from build123d import *

# Parameters (mm, degrees)
F0_W     = 140
F0_H     = 34.5
F1_DEPTH = 96
F2_W     = 140
F2_H     = 14.5
F3_DEPTH = 88
F4_W     = 1.7
F4_H     = 35.4929193519
F4_W_2   = 15.0318985057
F4_H_2   = 10
F5_DEPTH = 88


with BuildPart() as f1:
    # F0 (on Top) → F1 (new body)
    with BuildSketch(Plane.XY):
        with Locations((41.4941184592, -5.2499999292)):
            Rectangle(F0_W, F0_H)
    extrude(amount=F1_DEPTH)

    # F2 (on face) → F3 (cut)
    with BuildSketch(Plane.XY.offset(96)):
        with Locations((41.4941184592, -5.2499999292)):
            Rectangle(F2_W, F2_H)
    extrude(amount=-F3_DEPTH, mode=Mode.SUBTRACT)

    # F4 (on face) → F5 (cut)
    with BuildSketch(Plane.XY.offset(96)):
        Polygon((-13.0666754805, 12.0000000708), (-15.4708385365, 12.0000000708), (20.0220808154, -23.4929192811), (22.4262438715, -23.4929192811), align=None)
        Polygon((81.1649545925, 12.0000000708), (78.7607915364, 12.0000000708), (42.6027141511, -24.1580773145), (45.0068772072, -24.1580773145), align=None)
        with Locations((33.3644790113, -5.7464596052)):
            Rectangle(F4_W, F4_H)
        with Locations((103.9781692064, 7.0000000708)):
            Rectangle(F4_W_2, F4_H_2)
    extrude(amount=-F5_DEPTH, mode=Mode.SUBTRACT)


solid = f1.part
Verification items for the finished model (mm, model axes). A direction names the side the tool comes from. Give positions to 0.01 mm unless a question says otherwise; leave off trailing zeros. Write each loop counter-clockwise with the first axis right and the second up, starting at its lowest first coordinate (ties: lowest second). Pieces come first, ordered by that corner, then holes. Notation, with made-up numbers: (2, 31.5) - (39, 31.5) arc R14 ccw to (39, 56.5) - close; hole circle Ø5 at (62.25, 18.25). An arc over 180 degrees is marked (long way). Answer as CSV lines item,"result". Start each with the question number.
1. Draft check along X on faces 1 (the face through (9, 7, 96)), 2 (the face through (-7.997, 6.93, 52.616)). Enter one of: pulls with the +X half, pulls with the -X half, needs draft (parallel to the pull), parting line crosses it, or undercut.
2. Sectioned sample at C-C (y = 4.5). Record the boundary of the cut face in (x, z), then the cut area to 3 significant figures.
3. Thickness scan on line 1 (Y direction, x = 42, z = 73); line 2 (Y direction, x = 77, z = 87); line 3 (X direction, y = 5.5, z = 43.5). Record the ranges inside material, lowest first.
4. Sectioned sample at A-A (z = 28). Count the separate pieces of the cut face and the enclosed holes in it, then the cut area to 3 significant figures.
5. Set-up check for faces 3 (the face through (32.514, 7, 53)), 4 (the face through (51.595, -17.57, 52.616)), 5 (the face through (56, 7, 96)), 6 (the face through (84, -12.5, 53)), 7 (the face through (41, 12, 47)): record each of +Z, -Z, +X, -X, +Y, -Y from which the full face is reachable in a straight line by a thin tool's end or side.
6. Sectioned sample at D-D (x = 99.5). Record the boundary of the cut face in (y, z).
7. Depth check by flat-ended pin: pin 1 (3 mm diameter, centred on y = 4.5, z = 34, fed in from +X). Enter the tip coordinate at first touch or a pass-through.
8. Sectioned sample at B-B (x = 4). Record the boundary of the cut face in (y, z), then the cut area to 3 significant figures.
Derived:
1,face 1,"needs draft"
1,face 2,"undercut"
2,outline,"(-28.51, 0) - (111.49, 0) - (111.49, 8) - (96.46, 8) - (96.46, 96) - (73.66, 96) - (73.66, 8) - (71.26, 8) - (71.26, 96) - (34.21, 96) - (34.21, 8) - (32.51, 8) - (32.51, 96) - (-5.57, 96) - (-5.57, 8) - (-7.97, 8) - (-7.97, 96) - (-28.51, 96) - close"
2,area,"11,500 mm²"
3,line 1,"-22.5 to -12.5, 2 to 12"
3,line 2,"-22.5 to -12.5, 2 to 7.84, 10.24 to 12"
3,line 3,"-28.51 to -8.97, -6.57 to 32.51, 34.21 to 72.26, 74.66 to 96.46"
4,separate pieces,"8"
4,enclosed holes,"0"
4,area,"2,520 mm²"
5,face 3,"+Z, +Y, -Y"
5,face 4,"+Z"
5,face 5,"+Z, +X, -X, +Y, -Y"
5,face 6,"+Z, +X, -X"
5,face 7,"+Z, -Z, +X, -X, +Y"
6,outline,"(-22.5, 0) - (12, 0) - (12, 8) - (-12.5, 8) - (-12.5, 96) - (-22.5, 96) - close"
7,pin 1,"x = 96.46"
8,outline,"(-22.5, 0) - (12, 0) - (12, 96) - (2, 96) - (2, 8) - (-12.5, 8) - (-12.5, 96) - (-22.5, 96) - close"
8,area,"2,040 mm²"
